```python
from build123d import *

# Parameters (mm, degrees)
BOSS_EXTRU_1_DEPTH = 11
CONG_1_R           = 1


with BuildPart() as part:
    # Esquisse1 → Boss.-Extru.1 (new, symmetric)
    with BuildSketch(Plane.XY):
        with BuildLine():
            Line((-3, 0), (-6, 0))
            ThreePointArc((-6, 0), (-5.08732356, 5.980413612), (-2.432384342, 11.416370107))
            ThreePointArc((-2.432384342, 11.416370107), (-0.284041968, 13.314989212), (2.5, 14))
            Line((2.5, 14), (2.5, 1.658312395))
            ThreePointArc((2.5, 1.658312395), (-0.866025404, 2.872281323), (-3, 0))
        make_face()
    extrude(amount=BOSS_EXTRU_1_DEPTH, both=True)

    # Esquisse2 → Enlèvement de matière-Révolution1 (revolve, cut)
    with BuildSketch(Plane.XY, mode=Mode.PRIVATE) as enl_vement_de_mati_re_r_volution1_sk:
        Polygon((2.5, 7.5), (-1.5, 7.5), (-1.5, 6), (-5.081191808, 6), (-5.081191808, 9), (2.5, 9), align=None)
    revolve(enl_vement_de_mati_re_r_volution1_sk.sketch.rotate(Axis((-5.081191808, 9, 0), (-1, 0, 0)), 180), axis=Axis((-5.081191808, 9, 0), (-1, 0, 0)), mode=Mode.SUBTRACT)

    # Congé1
    cong_1_edges = [part.edges().sort_by_distance(p)[0] for p in [
        (-0.284041968, 13.314989212, 11),
        (-5.08732356, 5.980413612, 11),
        (-5.08732356, 5.980413612, -11),
        (-0.284041968, 13.314989212, -11),
        (2.5, 7.829156198, -11),
        (2.5, 7.829156198, 11),
        (2.5, 14, 0),
    ]]
    fillet(cong_1_edges, radius=CONG_1_R)

    # Symétrie1: part across plane


with BuildPart() as part_1:
    add(part.part)
    add(part.part.mirror(Plane(origin=(-3, 0, 11), x_dir=(0, 0, 1), z_dir=(0, 1, 0))))


solid = part_1.part
```
Build history of the part. All positions in model axes, mm. A direction names the side the tool comes from. Coordinates: 2 decimals unless noted, no trailing zeros. Write each loop counter-clockwise with the first axis right and the second up, starting at its lowest first coordinate (ties: lowest second). Pieces come first, ordered by that corner, then holes.
1. 3-axis set-ups, long thin cutter, end or side, ignore diameter. For faces 1 (the cylindrical face through (0.47, -7.5, -0.07)), 2 (the cylindrical face through (-3, -6, 0)): which of +Z, -Z, +X, -X, +Y, -Y reach the whole face in a straight line?
Answer block:
face 1: +X, -X
face 2: -X
2. Drill centre lines: probe 1 along Z at (x, y) = (0.8, -9); probe 2 along Z at (x, y) = (-2, -9); probe 3 along Y at (x, z) = (0, 5.75). Where is each one in solid material? Low to high.
Answer block:
probe 1: z = -11 to -1.5, 1.5 to 11
probe 2: z = -11 to -3, 3 to 11
probe 3: y = -13.45 to -3, 3 to 13.45
3. Pull direction Z, two halves, no side cores. Call faces 3 (the cylindrical face through (2.199, -7.2, 10.715)), 4 (the flat face through (-3.15, -0.18, -11)), 5 (the flat face through (-1.5, 7.7, 1.3)), 6 (the flat face through (-1.5, -7.7, 1.3)): released by +Z, released by -Z, zero draft, split by the parting line, or undercut.
Answer block:
face 3: released by +Z
face 4: released by -Z
face 5: undercut
face 6: undercut
4. Band-saw the part on B-B, the plane z = 4. Give the cut face in (x, y), and give its area (3 significant figures).
Answer block:
outline: (-2.43, -11.42) arc R6 ccw to (1.3, -13.88) arc R1 ccw to (2.5, -12.9) - (2.5, -1.66) arc R3 cw (long way) to (2.5, 1.66) - (2.5, 12.9) arc R1 ccw to (1.3, 13.88) arc R6 ccw to (-2.43, 11.42) arc R20.05 ccw to start
area: 158 mm2
5. Drop flat-ended pins along their axis: pin 1 (5 mm diameter, centred on x = 1, z = 3, fed in from -Y); pin 2 (2.5 mm diameter, centred on y = 9, z = 0, fed in from -X); pin 3 (8 mm diameter, centred on y = 4.5, z = 6, fed in from -X); pin 4 (1.8 mm diameter, centred on y = 10.5, z = 1, fed in from -X). Give the stop position or say it passes through.
Answer block:
pin 1: stops at y = -13.9
pin 2: passes through
pin 3: stops at x = -5.99
pin 4: stops at x = -1.5
6. Band-saw the part on A-A, the plane z = 0.75. Give the cut face in (x, y).
Answer block:
outline: (-5.05, -6.1) - (-1.5, -6.1) - (-1.5, -7.7) - (2.5, -7.7) - (2.5, -1.66) arc R3 cw (long way) to (2.5, 1.66) - (2.5, 7.7) - (-1.5, 7.7) - (-1.5, 6.1) - (-5.05, 6.1) arc R20.05 ccw to start; (-2.06, -11.9) arc R6 ccw to (1.3, -13.88) arc R1 ccw to (2.5, -12.9) - (2.5, -10.3) - (-1.5, -10.3) - (-1.5, -11.9) - close; (-2.06, 11.9) - (-1.5, 11.9) - (-1.5, 10.3) - (2.5, 10.3) - (2.5, 12.9) arc R1 ccw to (1.3, 13.88) arc R6 ccw to start
